Check sheet for the drawn part. Datum: minimum x, y, z corner. Units: mm. Give positions to 0.01 mm unless a question says otherwise; leave off trailing zeros. Loops run counter-clockwise (first coordinate to the right, second up) from the corner with the lowest first, then second, coordinate; pieces in that order, holes last. Notation, with made-up numbers: (10, 15) - (69, 15) arc R34 ccw to (69, 47) - close; hole circle Ø2 at (73.25, 37). An arc over 180 degrees is marked (long way). Use a Markdown table: item, result. Add a question column.
1. Material ranges on L1, parallel to Z at x = 4.8, y = 35.5; L2, parallel to X at y = 11.5, z = 32.5; L3, parallel to Y at x = 2, z = 29.5, recorded low to high.
2. Cross-section at C-C on y = 11. Enter the section's corners in (x, z), and give its area (3 significant figures).
3. Draft check along Y on the marked faces 1 and 2. Enter one of: pulls with the +Y half, pulls with the -Y half, needs draft (parallel to the pull), parting line crosses it, or undercut.
4. Depth check by flat-ended pin: P1, Ø7.5, axis at y = 10.39, z = 21, coming from the -X side; P2, Ø1.5, axis at x = 3, z = 8, coming from the -Y side; P3, Ø1.5, axis at x = 1, z = 50.5, coming from the +Y side. Enter the tip coordinate at first touch or a pass-through.
5. Cross-section at A-A on z = 35.5. Enter the section's corners in (x, y).
6. Cross-section at B-B on y = 35.5. Enter the section's corners in (x, z), and give its area (3 significant figures).
7. Cross-section at D-D on y = 50.5. Enter the section's corners in (x, z) (1 decimal).
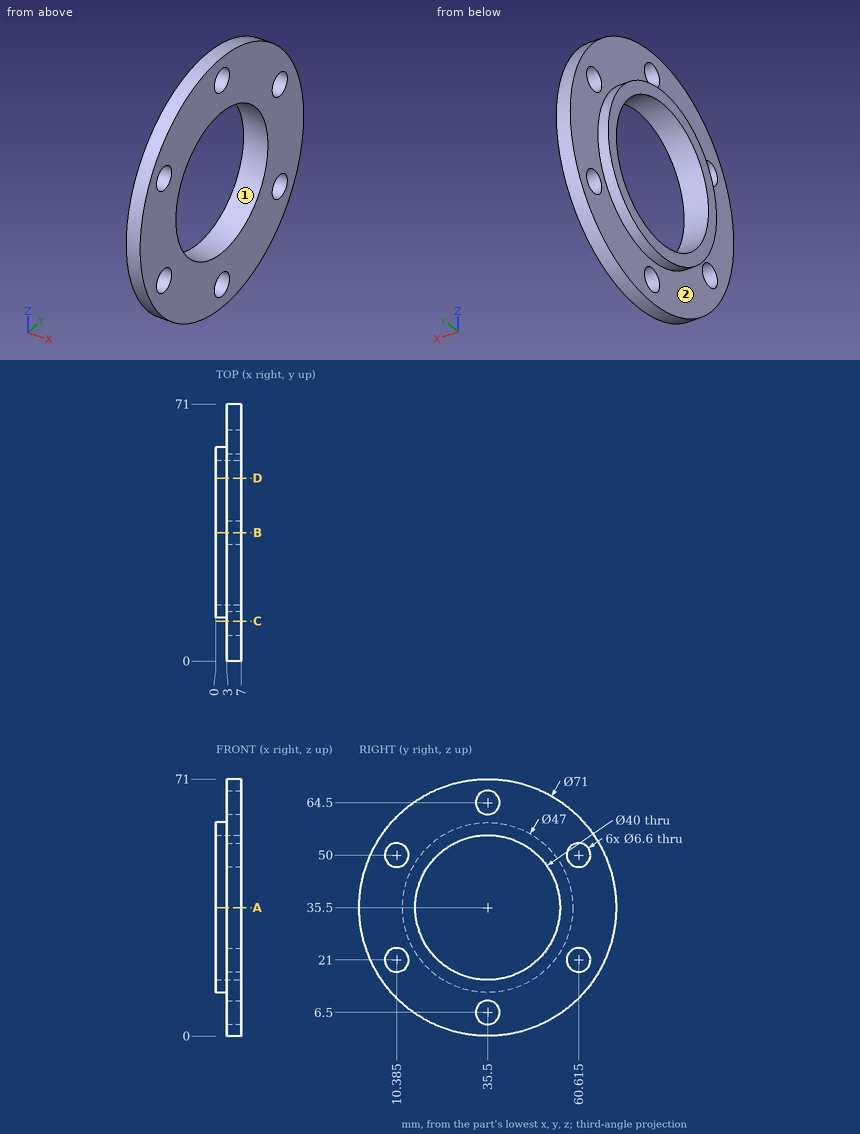
Values found:
| question | item | result |
|---|---|---|
| 1 | L1 | z = 0 to 3.2, 9.8 to 15.5, 55.5 to 61.2, 67.8 to 71 |
| 1 | L2 | x = 3 to 7 |
| 1 | L3 | y = 12.78 to 16.42, 54.58 to 58.22 |
| 2 | outline | (3, 9.81) - (7, 9.81) - (7, 17.76) - (3, 17.76) - close; (3, 24.24) - (7, 24.24) - (7, 46.76) - (3, 46.76) - close; (3, 53.24) - (7, 53.24) - (7, 61.19) - (3, 61.19) - close |
| 2 | area | 154 mm2 |
| 3 | face 1 | undercut |
| 3 | face 2 | needs draft |
| 4 | P1 | stops at x = 3 |
| 4 | P2 | stops at y = 12.16 |
| 4 | P3 | stops at y = 54.19 |
| 5 | outline | (0, 12) - (3, 12) - (3, 0) - (7, 0) - (7, 15.5) - (0, 15.5) - close; (0, 55.5) - (7, 55.5) - (7, 71) - (3, 71) - (3, 59) - (0, 59) - close |
| 6 | outline | (0, 12) - (3, 12) - (3, 9.8) - (7, 9.8) - (7, 15.5) - (0, 15.5) - close; (0, 55.5) - (7, 55.5) - (7, 61.2) - (3, 61.2) - (3, 59) - (0, 59) - close; (3, 0) - (7, 0) - (7, 3.2) - (3, 3.2) - close; (3, 67.8) - (7, 67.8) - (7, 71) - (3, 71) - close |
| 6 | area | 92.2 mm2 |
| 7 | outline | (0, 17.4) - (3, 17.4) - (3, 3.3) - (7, 3.3) - (7, 22.3) - (0, 22.3) - close; (0, 48.7) - (7, 48.7) - (7, 67.7) - (3, 67.7) - (3, 53.6) - (0, 53.6) - close |
